Verification items for this drawing (mm, ordinates from the low corner). A direction names the side the tool comes from. Give positions to 0.01 mm unless a question says otherwise; leave off trailing zeros. Write each loop counter-clockwise with the first axis right and the second up, starting at its lowest first coordinate (ties: lowest second). Pieces come first, ordered by that corner, then holes. Notation, with made-up numbers: (-39, -3) -> (-20, -3) arc R10 cw to (-20, 2) -> close; hole circle Ø9 at (15, 16). An arc over 180 degrees is marked (long way). Use one line per item in the form item = value. Start each with the question number.
(1) Scan lines: L1, parallel to Y at x = 1.2, z = 55.5; L2, parallel to X at y = 8, z = 45; L3, parallel to Z at x = 2, y = 7. Record each from-to range of solid material in increasing order.
(2) Depth check by flat-ended pin: pin 1 Ø2 at (x, z) = (29.5, 40) entering from +Y; pin 2 Ø4.5 at (x, y) = (1.5, 12) entering from -Z. Enter the tip coordinate at first touch or a pass-through.
(3) Set-up check for the marked faces 5 and 6: record each of +Z, -Z, +X, -X, +Y, -Y from which the full face is reachable in a straight line by a thin tool's end or side.
(4) Section check C-C, the plane x = 6. Record the cut outline in (y, z), plus the area to 3 significant figures.
(5) Section check B-B, the plane y = 7.5. Record the cut outline in (x, z), plus the area to 3 significant figures.
(6) Section check D-D, the plane z = 55.5. Record the cut outline in (x, y), plus the area to 3 significant figures.
(7) Section check A-A, the plane x = 22. Record the cut outline in (y, z).
(8) Release check for a two-part mould opening along X. For the marked faces 1, 2, 3 and 4 record: pulls with the +X half, pulls with the -X half, needs draft (parallel to the pull), parting line crosses it, or undercut.
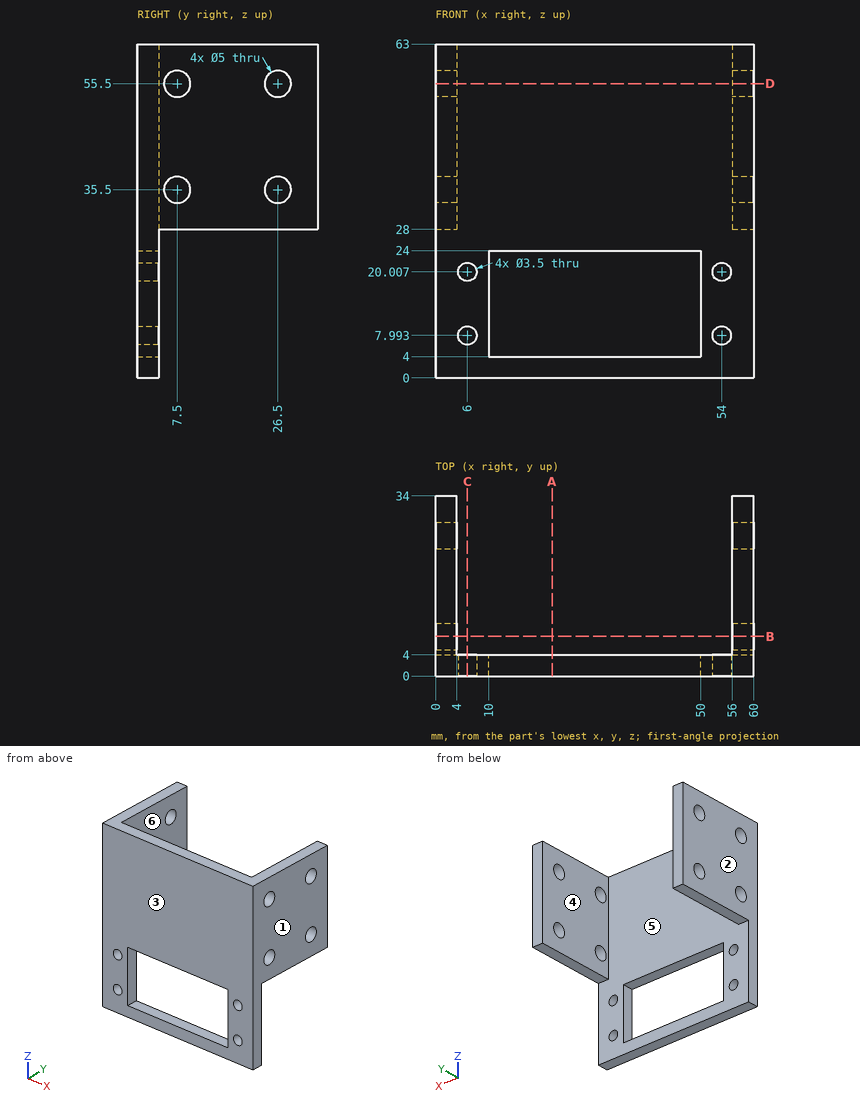
Completed:
q1.L1 = 0 to 5, 10 to 24, 29 to 34
q1.L2 = 0 to 4, 56 to 60
q1.L3 = 28 to 33.05, 37.95 to 53.05, 57.95 to 63
q2.pin_1 = 4
q2.pin_2 = 28
q3.face_5 = -Z, +Y
q3.face_6 = +Z, -Z, +Y
q4.outline = (0, 0) -> (4, 0) -> (4, 6.24) -> (0, 6.24) -> close; (0, 9.74) -> (4, 9.74) -> (4, 18.26) -> (0, 18.26) -> close; (0, 21.76) -> (4, 21.76) -> (4, 63) -> (0, 63) -> close
q4.area = 224 mm²
q5.outline = (0, 28) -> (4, 28) -> (4, 33) -> (0, 33) -> close; (0, 38) -> (4, 38) -> (4, 53) -> (0, 53) -> close; (0, 58) -> (4, 58) -> (4, 63) -> (0, 63) -> close; (56, 28) -> (60, 28) -> (60, 33) -> (56, 33) -> close; (56, 38) -> (60, 38) -> (60, 53) -> (56, 53) -> close; (56, 58) -> (60, 58) -> (60, 63) -> (56, 63) -> close
q5.area = 200 mm²
q6.outline = (0, 0) -> (60, 0) -> (60, 5) -> (56, 5) -> (56, 4) -> (4, 4) -> (4, 5) -> (0, 5) -> close; (0, 10) -> (4, 10) -> (4, 24) -> (0, 24) -> close; (0, 29) -> (4, 29) -> (4, 34) -> (0, 34) -> close; (56, 10) -> (60, 10) -> (60, 24) -> (56, 24) -> close; (56, 29) -> (60, 29) -> (60, 34) -> (56, 34) -> close
q6.area = 400 mm²
q7.outline = (0, 0) -> (4, 0) -> (4, 4) -> (0, 4) -> close; (0, 24) -> (4, 24) -> (4, 63) -> (0, 63) -> close
q8.face_1 = pulls with the +X half
q8.face_2 = pulls with the -X half
q8.face_3 = needs draft
q8.face_4 = undercut
